from build123d import *

# Parameters (mm, degrees)
SKETCH1_W           = 66
SKETCH1_H           = 16
SKETCH1_R           = 1.5
BOSS_EXTRUDE1_DEPTH = 1.5
SKETCH2_W           = 2.5
SKETCH2_H           = 2.5
BOSS_EXTRUDE2_DEPTH = 2.54
SKETCH3_W           = 0.64
SKETCH3_H           = 0.64
BOSS_EXTRUDE3_DEPTH = 6
LPATTERN1_COUNT     = 6
LPATTERN1_PITCH     = 2.54
LPATTERN1_COL_COUNT = 6
LPATTERN1_COL_PITCH = 2.54
SKETCH4_W           = 2.7
SKETCH4_H           = 3.35
BOSS_EXTRUDE4_DEPTH = 1.6


with BuildPart() as part:
    # Sketch1 → Boss-Extrude1 (new body)
    with BuildSketch(Plane(origin=(0, 0, 0), x_dir=(1, 0, 0), z_dir=(0, 1, 0))):
        Rectangle(SKETCH1_W, SKETCH1_H)
        with Locations((-18, -4.5)):
            Circle(SKETCH1_R, mode=Mode.SUBTRACT)
        with Locations((18, -4.5)):
            Circle(SKETCH1_R, mode=Mode.SUBTRACT)
    extrude(amount=-BOSS_EXTRUDE1_DEPTH)

    # Sketch2 → Boss-Extrude2 (add)
    with BuildSketch(Plane.XZ.offset(1.5)):
        with Locations((0, 6.73)):
            Rectangle(SKETCH2_W, SKETCH2_H)
    boss_extrude2 = extrude(amount=BOSS_EXTRUDE2_DEPTH)

    # Sketch3 → Boss-Extrude3 (add)
    with BuildSketch(Plane(origin=(0, -4.04, 0), x_dir=(-1, 0, 0), z_dir=(0, -1, 0))):
        with Locations((0, -6.73)):
            Rectangle(SKETCH3_W, SKETCH3_H)
    boss_extrude3 = extrude(amount=BOSS_EXTRUDE3_DEPTH)

    # LPattern1: Boss-Extrude2, Boss-Extrude3 ×6
    with Locations(*[(-i * LPATTERN1_PITCH, 0, 0) for i in range(1, LPATTERN1_COUNT)]):
        add(boss_extrude2)
        add(boss_extrude3)

    # LPattern1 col: Boss-Extrude2, Boss-Extrude3 ×6
    with Locations(*[(i * LPATTERN1_COL_PITCH, 0, 0) for i in range(1, LPATTERN1_COL_COUNT)]):
        add(boss_extrude2)
        add(boss_extrude3)

    # Sketch4 → Boss-Extrude4 (add)
    with BuildSketch(Plane(origin=(0, 0, 0), x_dir=(1, 0, 0), z_dir=(0, 1, 0))):
        with Locations((-4.1, 5.425)):
            Rectangle(SKETCH4_W, SKETCH4_H)
        with Locations((4.1, 5.425)):
            Rectangle(SKETCH4_W, SKETCH4_H)
        with Locations((12.3, 5.425)):
            Rectangle(SKETCH4_W, SKETCH4_H)
        with Locations((20.5, 5.425)):
            Rectangle(SKETCH4_W, SKETCH4_H)
        with Locations((28.7, 5.425)):
            Rectangle(SKETCH4_W, SKETCH4_H)
        with Locations((-12.3, 5.425)):
            Rectangle(SKETCH4_W, SKETCH4_H)
        with Locations((-28.7, 5.425)):
            Rectangle(SKETCH4_W, SKETCH4_H)
        with Locations((-20.5, 5.425)):
            Rectangle(SKETCH4_W, SKETCH4_H)
    extrude(amount=BOSS_EXTRUDE4_DEPTH)


solid = part.part
Geometry check sheet. Reference: the model listing, model coordinates, mm. A direction names the side the tool comes from. Round coordinates to 2 decimals unless told otherwise and drop trailing zeros. Loops run counter-clockwise (first coordinate to the right, second up) from the corner with the lowest first, then second, coordinate; pieces in that order, holes last.
Item 1: Cross-section at C-C on z = 4.5. Record the boundary of the cut face in (x, y), then the cut area to 3 significant figures.
Item 2: Cross-section at B-B on x = 18. Record the boundary of the cut face in (y, z), then the cut area to 3 significant figures.
Item 3: Thickness scan on line 1 (X direction, y = -0.7, z = 4.5); line 2 (Z direction, x = -18, y = -0.9); line 3 (Y direction, x = 4, z = 2). Record the ranges inside material, lowest first.
Item 4: Cross-section at A-A on y = 0.75. Count the separate pieces of the cut face and the enclosed holes in it, then the cut area to 3 significant figures.
Item 5: Gauge pin test, flat ends, axial feed: pin 1 (1.2 mm diameter, centred on y = -2.5, z = 7.5, fed in from -X); pin 2 (1 mm diameter, centred on x = -15, y = -7, fed in from -Z); pin 3 (2 mm diameter, centred on x = 3, y = -3, fed in from -Z); pin 4 (0.5 mm diameter, centred on y = 0.5, z = -5, fed in from -X). Record the tip position at first contact, or that the pin passes through.
Item 6: Access from +Z, -Z, +X, -X, +Y, -Y to the whole of each face (thin tool, end or side, straight path). Record for faces 1 (the flat face through (-21, 1.6, -5)), 2 (the flat face through (-19.15, 1, -5)), 3 (the flat face through (30.05, 1, -5)), 4 (the flat face through (10, -3, 5.48)).
Answer sheet:
1. outline: (-33, -1.5) - (-19.5, -1.5) - (-19.5, 0) - (-33, 0) - close; (-16.5, -1.5) - (16.5, -1.5) - (16.5, 0) - (-16.5, 0) - close; (19.5, -1.5) - (33, -1.5) - (33, 0) - (19.5, 0) - close
1. area: 90.0 mm2
2. outline: (-1.5, -8) - (0, -8) - (0, 3) - (-1.5, 3) - close; (-1.5, 6) - (0, 6) - (0, 8) - (-1.5, 8) - close
2. area: 19.5 mm2
3. line 1: x = -33 to -19.5, -16.5 to 16.5, 19.5 to 33
3. line 2: z = -8 to 3, 6 to 8
3. line 3: y = -1.5 to 0
4. separate pieces: 8
4. enclosed holes: 0
4. area: 72.4 mm2
5. pin 1: stops at x = -13.95
5. pin 2: passes through
5. pin 3: stops at z = 5.48
5. pin 4: stops at x = -30.05
6. face 1: +Z, -Z, +X, -X, +Y
6. face 2: +Z, -Z, +Y
6. face 3: +Z, -Z, +X, +Y
6. face 4: -Z, +X, -X, -Y
